from build123d import *

# Parameters (mm, degrees)
ESQUISSE1_W             = 54.7
ESQUISSE1_H             = 30
EXTRUSION1_DEPTH        = 5
ESQUISSE2_R             = 1.5
ENL_V_MAT_EXTRU_1_DEPTH = 54.806040553
ESQUISSE3_R             = 2.9
ENL_V_MAT_EXTRU_2_DEPTH = 54.641215497
ESQUISSE4_R             = 1.5
ENL_V_MAT_EXTRU_3_DEPTH = 54.806040553


with BuildPart() as part:
    # Esquisse1 → Extrusion1 (new body)
    with BuildSketch(Plane(origin=(0, 0, 0), x_dir=(1, 0, 0), z_dir=(0, 1, 0))):
        with Locations((-22.35, 5)):
            Rectangle(ESQUISSE1_W, ESQUISSE1_H)
    extrude(amount=EXTRUSION1_DEPTH)

    # Esquisse2 → Enlèv. mat.-Extru.1 (cut, through all)
    with BuildSketch(Plane(origin=(0, 5, 0), x_dir=(1, 0, 0), z_dir=(0, 1, 0))):
        with Locations(Location((-16, 0, 0), (0, 0, 270))):
            Circle(ESQUISSE2_R)
    extrude(amount=-ENL_V_MAT_EXTRU_1_DEPTH, mode=Mode.SUBTRACT)

    # Esquisse3 → Enlèv. mat.-Extru.2 (cut, through all)
    with BuildSketch(Plane.XZ.offset(-2.3)):
        with Locations((-16, 0)):
            Circle(ESQUISSE3_R)
    extrude(amount=-ENL_V_MAT_EXTRU_2_DEPTH, mode=Mode.SUBTRACT)

    # Esquisse4 → Enlèv. mat.-Extru.3 (cut, through all)
    with BuildSketch(Plane(origin=(0, 5, 0), x_dir=(1, 0, 0), z_dir=(0, 1, 0))):
        with Locations(Location((2.5, -6, 0), (0, 0, 270))):
            Circle(ESQUISSE4_R)
        with Locations(Location((2.5, 16, 0), (0, 0, 270))):
            Circle(ESQUISSE4_R)
        with Locations(Location((-47.2, 16, 0), (0, 0, 270))):
            Circle(ESQUISSE4_R)
        with Locations(Location((-47.2, -6, 0), (0, 0, 270))):
            Circle(ESQUISSE4_R)
    extrude(amount=-ENL_V_MAT_EXTRU_3_DEPTH, mode=Mode.SUBTRACT)


solid = part.part
Read the model definition and answer for the solid it produces. Units are mm, in the model's axes. A direction names the side the tool comes from. Give positions to 0.01 mm unless a question says otherwise; leave off trailing zeros. Loops run counter-clockwise (first coordinate to the right, second up) from the corner with the lowest first, then second, coordinate; pieces in that order, holes last. Notation, with made-up numbers: (-15, 77.25) -> (19, 77.25) arc R35 cw to (19, 116.25) -> close; hole circle Ø2 at (24.5, 8). An arc over 180 degrees is marked (long way). Answer as CSV lines item,"result".
Item 1: Find section C-C on x = -16. Give the vertices of the cut face in (y, z), plus the area to 3 significant figures.
Returned:
outline,"(0, -20) -> (5, -20) -> (5, -2.9) -> (2.3, -2.9) -> (2.3, -1.5) -> (0, -1.5) -> close; (0, 1.5) -> (2.3, 1.5) -> (2.3, 2.9) -> (5, 2.9) -> (5, 10) -> (0, 10) -> close"
area,"127 mm²"
Item 2: Find section B-B on z = 0. Give the vertices of the cut face in (x, y), plus the area to 3 significant figures.
Returned:
outline,"(-49.7, 0) -> (-17.5, 0) -> (-17.5, 2.3) -> (-18.9, 2.3) -> (-18.9, 5) -> (-49.7, 5) -> close; (-14.5, 0) -> (5, 0) -> (5, 5) -> (-13.1, 5) -> (-13.1, 2.3) -> (-14.5, 2.3) -> close"
area,"251 mm²"
Item 3: Find section A-A on x = -47.2. Give the vertices of the cut face in (y, z), plus the area to 3 significant figures.
Returned:
outline,"(0, -20) -> (5, -20) -> (5, -17.5) -> (0, -17.5) -> close; (0, -14.5) -> (5, -14.5) -> (5, 4.5) -> (0, 4.5) -> close; (0, 7.5) -> (5, 7.5) -> (5, 10) -> (0, 10) -> close"
area,"120 mm²"
Item 4: For faces 1 (the face through (-23, 0, -5)), 2 (the face through (-18.9, 3.6, 0.1)), determine the directions among +Z, -Z, +X, -X, +Y, -Y from which every point of the face is accessible in a straight line to the end or side of a thin tool.
Returned:
face 1,"+Z, -Z, +X, -X, -Y"
face 2,"+Y"
Item 5: Find section D-D on y = 2.95. Give the vertices of the cut face in (x, z), plus the area to 3 significant figures.
Returned:
outline,"(-49.7, -20) -> (5, -20) -> (5, 10) -> (-49.7, 10) -> close; hole circle Ø3 at (-47.2, -16); hole circle Ø3 at (-47.2, 6); hole circle Ø5.8 at (-16, 0); hole circle Ø3 at (2.5, -16); hole circle Ø3 at (2.5, 6)"
area,"1,590 mm²"
Item 6: This flat-tipped pin is pushed along its axis until it touches: pin 1 (3 mm diameter, centred on x = -15, z = 0, fed in from +Y). Where does it stop, or does it pass through?
Returned:
pin 1,"stops at y = 2.3"
Item 7: Consider line 1 (X direction, y = 1.8, z = 6); line 2 (X direction, y = 2.5, z = -15.5); line 3 (Z direction, x = -16, y = 2.95). Determine where each line is inside the solid, lowest interval first. Write a range as [from, to].
Returned:
line 1,"x = [-49.7, -48.7], [-45.7, 1], [4, 5]"
line 2,"x = [-49.7, -48.61], [-45.79, 1.09], [3.91, 5]"
line 3,"z = [-20, -2.9], [2.9, 10]"
Item 8: Determine the mould class of faces 3 (the face through (1.6, 2.5, 4.8)), 4 (the face through (-46.19, 2.54, 4.89)), 5 (the face through (-23, 2, -20)), 6 (the face through (-23, 5, -5)) for opening direction Z: +Z half, -Z half, draft (parallel to the pull), parting line (faces both ways), or undercut.
Returned:
face 3,"undercut"
face 4,"undercut"
face 5,"-Z half"
face 6,"draft"
